```python
from build123d import *

# Parameters (mm, degrees)
F0_W     = 2
F0_H     = 1.5
F1_DEPTH = 5.2
F2_DEPTH = 3.7
F3_DEPTH = 3.9
F4_R     = 0.2


with BuildPart() as f1:
    # F0 (on Front) → F1 (new body, symmetric)
    with BuildSketch(Plane.XZ):
        Polygon((-4.75, 4.25), (9.75, 4.25), (9.75, 5.75), (6.75, 5.75), (2.5, 5.75), (-4.75, 5.75), align=None)
        Polygon((2.5, 5.75), (6.75, 5.75), (6.75, 8), (4.75, 8), align=None)
        Polygon((6.75, -5.75), (9.75, -5.75), (9.75, -4.75), (-8.75, -4.75), (-8.75, 4.25), (-6.75, 4.25), (-6.75, 5.75), (-9.75, 5.75), (-9.75, -5.75), (2.5, -5.75), align=None)
        Polygon((6.75, -8), (6.75, -5.75), (2.5, -5.75), (4.75, -8), align=None)
        Polygon((-8.75, -4.75), (9.75, -4.75), (9.75, 4.25), (-4.75, 4.25), (-6.75, 4.25), (-8.75, 4.25), align=None)
        with Locations((-5.75, 5)):
            Rectangle(F0_W, F0_H)
    extrude(amount=F1_DEPTH, both=True)

    # F0 (on Front) → F2 (cut, symmetric)
    with BuildSketch(Plane.XZ):
        with Locations((-5.75, 5)):
            Rectangle(F0_W, F0_H)
    extrude(amount=F2_DEPTH, both=True, mode=Mode.SUBTRACT)

    # F0 (on Front) → F3 (cut, symmetric)
    with BuildSketch(Plane.XZ):
        Polygon((-8.75, -4.75), (9.75, -4.75), (9.75, 4.25), (-4.75, 4.25), (-6.75, 4.25), (-8.75, 4.25), align=None)
    extrude(amount=F3_DEPTH, both=True, mode=Mode.SUBTRACT)

    # F4
    f4_edges = [f1.edges().sort_by_distance(p)[0] for p in [
        (-3.625, -5.2, 5.75),
        (3.625, -5.2, 6.875),
        (6.75, 0, 8),
        (4.75, 0, 8),
        (5.75, -5.2, 8),
        (6.75, -5.2, 6.875),
        (8.25, -5.2, 5.75),
        (8.25, 5.2, 5.75),
        (-3.625, 5.2, 5.75),
        (3.625, 5.2, 6.875),
        (5.75, 5.2, 8),
        (-9.75, 0, 5.75),
        (-9.75, -5.2, 0),
        (-3.625, -5.2, -5.75),
        (5.75, -5.2, -8),
        (8.25, -5.2, -5.75),
        (6.75, 0, -8),
        (4.75, 0, -8),
        (3.625, 5.2, -6.875),
        (3.625, -5.2, -6.875),
        (5.75, 5.2, -8),
        (-3.625, 5.2, -5.75),
        (8.25, 5.2, -5.75),
        (6.75, 5.2, -6.875),
        (-9.75, 5.2, 0),
        (-9.75, 0, -5.75),
        (6.75, 5.2, 6.875),
        (6.75, -5.2, -6.875),
    ]]
    fillet(f4_edges, radius=F4_R)


solid = f1.part
```
Here's how the part is built. I have some questions about the finished solid (model axes, mm). A direction names the side the tool comes from. Round coordinates to 2 decimals unless told otherwise and drop trailing zeros. Loops run counter-clockwise (first coordinate to the right, second up) from the corner with the lowest first, then second, coordinate; pieces in that order, holes last. Notation, with made-up numbers: (-10, -18) -> (-3, -18) arc R33 cw to (-3, 17) -> close; hole circle Ø3 at (32, -35). An arc over 180 degrees is marked (long way). Answer as CSV lines item,"result". Start each with the question number.
1. If we mould it in two halves opening along X, with no side actions, what happens to faces 1 (the face through (-4, 0, -5.75)), 2 (the face through (-6.75, 0, 5)), 3 (the face through (6.75, 0, -7))? For each: pulls with the +X half, pulls with the -X half, needs draft (parallel to the pull), parting line crosses it, or undercut.
2. I need wall thicknesses on probe 1 along Z at (x, y) = (6.25, -3.75); probe 2 along Y at (x, z) = (-4.5, 2.5); probe 3 along Z at (x, y) = (-7, -3.5). Which ranges of each line are inside material? Lowest first, please. Write a range as from..to.
3. Imagine slicing it at D-D on x = -6. Write out the boundary of the cut face in (y, z).
4. Imagine slicing it at B-B on z = 2.25. Write out the boundary of the cut face in (x, y), plus the area to 3 significant figures.
5. I'm going to push flat-ended pins straight in: P1, Ø2.5, axis at x = 2.5, y = -0.5, coming from the +Z side; P2, Ø5, axis at x = -5.5, y = 2.5, coming from the +Z side; P3, Ø4, axis at x = 1.5, y = -2, coming from the -Z side. Where does each tip first touch, or does it pass through?
6. Imagine slicing it at A-A on y = 2.75. Write out the boundary of the cut face in (x, z), plus the area to 3 significant figures.
7. Imagine slicing it at C-C on x = 5.5. Write out the boundary of the cut face in (y, z), plus the area to 3 significant figures.
8. For faces 4 (the face through (8, 0, -5.75)), 5 (the face through (-6, -3.7, 5)), 6 (the face through (-3, 0, 5.75)), which set-ups out of +Z, -Z, +X, -X, +Y, -Y let a thin tool reach every point of the face, with its end or its side?
Solution:
1,face 1,"needs draft"
1,face 2,"undercut"
1,face 3,"pulls with the +X half"
2,probe 1,"-8..-4.75, 4.25..8"
2,probe 2,"-5.2..-3.9, 3.9..5.2"
2,probe 3,"-5.75..-4.75, 4.25..5.75"
3,outline,"(-5.2, -5.55) arc R0.2 ccw to (-5, -5.75) -> (5, -5.75) arc R0.2 ccw to (5.2, -5.55) -> (5.2, 5.55) arc R0.2 ccw to (5, 5.75) -> (3.7, 5.75) -> (3.7, 4.25) -> (3.9, 4.25) -> (3.9, -4.75) -> (-3.9, -4.75) -> (-3.9, 4.25) -> (-3.7, 4.25) -> (-3.7, 5.75) -> (-5, 5.75) arc R0.2 ccw to (-5.2, 5.55) -> close"
4,outline,"(-9.75, -5) arc R0.2 ccw to (-9.55, -5.2) -> (9.75, -5.2) -> (9.75, -3.9) -> (-8.75, -3.9) -> (-8.75, 3.9) -> (9.75, 3.9) -> (9.75, 5.2) -> (-9.55, 5.2) arc R0.2 ccw to (-9.75, 5) -> close"
4,area,"58.5 mm²"
5,P1,"z = 7"
5,P2,"z = 5.75"
5,P3,"z = -6.75"
6,outline,"(-9.75, -5.55) arc R0.2 ccw to (-9.55, -5.75) -> (2.5, -5.75) -> (4.69, -7.94) arc R0.2 ccw to (4.83, -8) -> (6.55, -8) arc R0.2 ccw to (6.75, -7.8) -> (6.75, -5.75) -> (9.75, -5.75) -> (9.75, -4.75) -> (-8.75, -4.75) -> (-8.75, 4.25) -> (-6.75, 4.25) -> (-6.75, 5.75) -> (-9.55, 5.75) arc R0.2 ccw to (-9.75, 5.55) -> close; (-4.75, 4.25) -> (9.75, 4.25) -> (9.75, 5.75) -> (6.75, 5.75) -> (6.75, 7.8) arc R0.2 ccw to (6.55, 8) -> (4.83, 8) arc R0.2 ccw to (4.69, 7.94) -> (2.5, 5.75) -> (-4.75, 5.75) -> close"
6,area,"68.8 mm²"
7,outline,"(-5.2, -7.8) arc R0.2 ccw to (-5, -8) -> (5, -8) arc R0.2 ccw to (5.2, -7.8) -> (5.2, 7.8) arc R0.2 ccw to (5, 8) -> (-5, 8) arc R0.2 ccw to (-5.2, 7.8) -> close; hole (-3.9, -4.75) -> (3.9, -4.75) -> (3.9, 4.25) -> (-3.9, 4.25) -> close"
7,area,"96.2 mm²"
8,face 4,"-Z, +X, +Y, -Y"
8,face 5,"+Z"
8,face 6,"+Z, -X, +Y, -Y"
